Verification items for this drawing (mm, ordinates from the low corner). A direction names the side the tool comes from. Round coordinates to 2 decimals unless told otherwise and drop trailing zeros. Write each loop counter-clockwise with the first axis right and the second up, starting at its lowest first coordinate (ties: lowest second). Pieces come first, ordered by that corner, then holes.
Item 1: Scan lines: probe 1 along Z at (x, y) = (17.5, 100.5); probe 2 along Y at (x, z) = (15.5, 111); probe 3 along Z at (x, y) = (6.75, 344.5). Record each from-to range of solid material in increasing order.
Item 2: Cross-section at A-A (x = 7.25). Enter the section's corners in (y, z), then the cut area to 3 significant figures.
Item 3: Depth check by flat-ended pin: P1, Ø9, axis at x = 12, y = 347.5, coming from the -Z side; P2, Ø10, axis at x = 7.5, y = 285.5, coming from the -Z side; P3, Ø5.5, axis at x = 13.5, z = 8, coming from the -Y side. Enter the tip coordinate at first touch or a pass-through.
Item 4: Cross-section at C-C (y = 332). Enter the section's corners in (x, z), then the cut area to 3 significant figures.
Item 5: Access from +Z, -Z, +X, -X, +Y, -Y to the whole of each face (thin tool, end or side, straight path). Record for the marked faces 1, 2 and 3.
Item 6: Cross-section at B-B (z = 106). Enter the section's corners in (x, y), then the cut area to 3 significant figures.
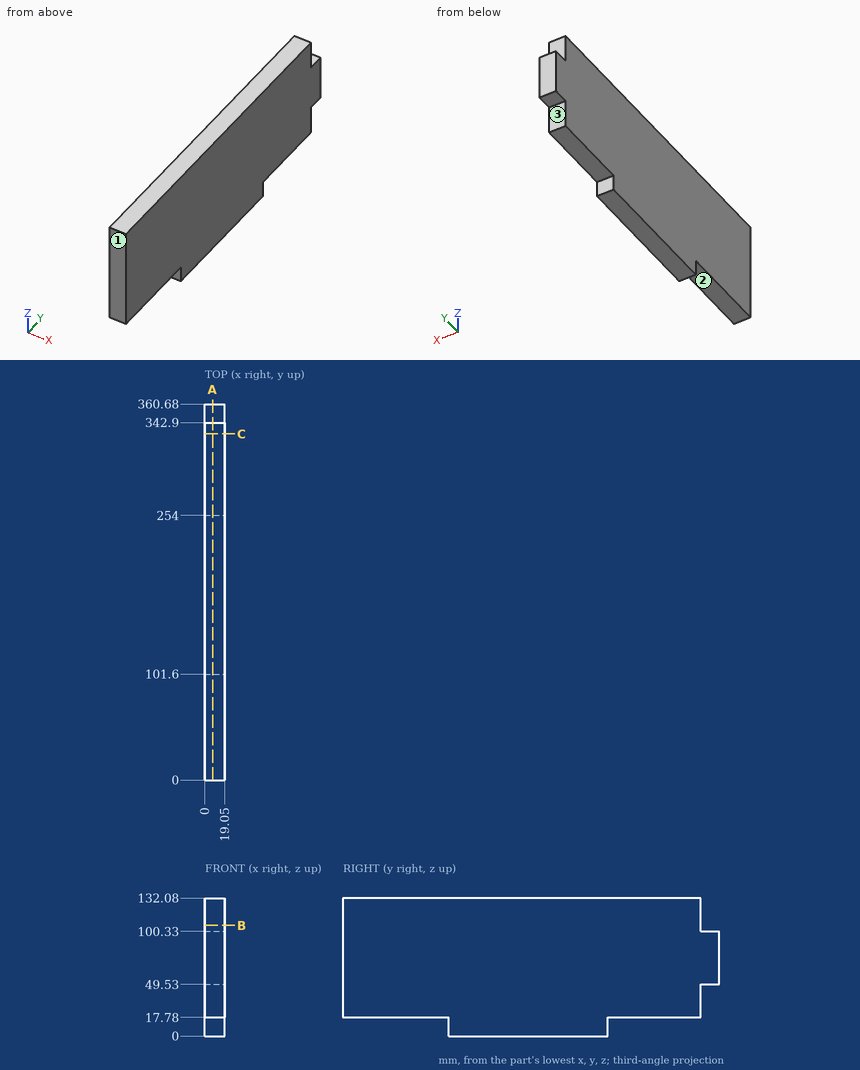
Resolved:
1. probe 1: z = 17.78 to 132.08
1. probe 2: y = 0 to 342.9
1. probe 3: z = 49.53 to 100.33
2. outline: (0, 17.78) - (101.6, 17.78) - (101.6, 0) - (254, 0) - (254, 17.78) - (342.9, 17.78) - (342.9, 49.53) - (360.68, 49.53) - (360.68, 100.33) - (342.9, 100.33) - (342.9, 132.08) - (0, 132.08) - close
2. area: 42,800 mm2
3. P1: stops at z = 49.53
3. P2: stops at z = 17.78
3. P3: stops at y = 101.6
4. outline: (0, 17.78) - (19.05, 17.78) - (19.05, 132.08) - (0, 132.08) - close
4. area: 2,180 mm2
5. face 1: +Z, -Z, +X, -X, -Y
5. face 2: -Z, +X, -X, -Y
5. face 3: -Z, +X, -X, +Y
6. outline: (0, 0) - (19.05, 0) - (19.05, 342.9) - (0, 342.9) - close
6. area: 6,530 mm2
